Input: part model. Units: mm. Frame: model coordinates. Give positions to 0.01 mm unless a question says otherwise; leave off trailing zeros. Loops run counter-clockwise (first coordinate to the right, second up) from the corner with the lowest first, then second, coordinate; pieces in that order, holes last. Notation, with made-up numbers: M -40,76.5 L 17,76.5 A18 cw 17,110.5 Z; hole C -5.5,-29 d7. An arc over 180 degrees is marked long. Use CSV: the item, a comma, the result in double quotes. Start each with the question number.
from build123d import *

# Parameters (mm, degrees)
BOSS_EXTRU_1_DEPTH = 0.7


with BuildPart() as part:
    # Esquisse1 → Boss.-Extru.1 (new body)
    with BuildSketch(Plane.XY.offset(0.7)):
        with BuildLine():
            Line((0.632886418, 2.207137237), (0.815865574, 2.845261388))
            ThreePointArc((0.815865574, 2.845261388), (1.110405111, 3.18363768), (1.558931601, 3.174917521))
            ThreePointArc((1.558931601, 3.174917521), (2.501036685, 2.501036685), (3.174917521, 1.558931601))
            ThreePointArc((3.174917521, 1.558931601), (3.18363768, 1.110405111), (2.845261388, 0.815865574))
            Line((2.845261388, 0.815865574), (2.207137237, 0.632886418))
            ThreePointArc((2.207137237, 0.632886418), (2.027919172, 0.500132947), (1.979974043, 0.282316824))
            ThreePointArc((1.979974043, 0.282316824), (1.989252382, -0.2070627), (1.879385242, -0.684040287))
            Line((1.879385242, -0.684040287), (2.561408424, -2.557883579))
            ThreePointArc((2.561408424, -2.557883579), (3.113603209, -3.004615598), (3.76702433, -2.726174553))
            ThreePointArc((3.76702433, -2.726174553), (0, 4.65), (-3.76702433, -2.726174553))
            ThreePointArc((-3.76702433, -2.726174553), (-3.113603209, -3.004615598), (-2.561408424, -2.557883579))
            Line((-2.561408424, -2.557883579), (-1.879385242, -0.684040287))
            ThreePointArc((-1.879385242, -0.684040287), (-1.989252382, -0.2070627), (-1.979974043, 0.282316824))
            ThreePointArc((-1.979974043, 0.282316824), (-2.027919172, 0.500132947), (-2.207137237, 0.632886418))
            Line((-2.207137237, 0.632886418), (-2.845261388, 0.815865574))
            ThreePointArc((-2.845261388, 0.815865574), (-3.18363768, 1.110405111), (-3.174917521, 1.558931601))
            ThreePointArc((-3.174917521, 1.558931601), (-2.501036685, 2.501036685), (-1.558931601, 3.174917521))
            ThreePointArc((-1.558931601, 3.174917521), (-1.110405111, 3.18363768), (-0.815865574, 2.845261388))
            Line((-0.815865574, 2.845261388), (-0.632886418, 2.207137237))
            ThreePointArc((-0.632886418, 2.207137237), (-0.500132947, 2.027919172), (-0.282316824, 1.979974043))
            ThreePointArc((-0.282316824, 1.979974043), (0, 2), (0.282316824, 1.979974043))
            ThreePointArc((0.282316824, 1.979974043), (0.500132947, 2.027919172), (0.632886418, 2.207137237))
        make_face()
    extrude(amount=-BOSS_EXTRU_1_DEPTH)


solid = part.part
Item 1: Section B-B (x = -3). Output: boundary loops of the cut face in (y, z).
Item 2: First-contact query: pin 1 Ø2 at (x, y) = (0, 2.5) entering from -Z. Flat tip, straight axial feed; report the tip coordinate or a pass-through.
Item 3: Section C-C (z = 0.1). Output: boundary loops of the cut face in (x, y).
Item 4: Section A-A (y = 0). Output: boundary loops of the cut face in (x, z).
Item 5: Mould query, pull axis X, two halves, no side actions, for faces 1 (the cylindrical face through (0.143, 4.648, 0.355)), 2 (the cylindrical face through (-2.5, 2.5, 0.4)), 3 (the cylindrical face through (2.5, 2.5, 0.4)), 4 (the flat face through (0, 3, 0.7)). Classes: +X half, -X half, draft (parallel to the pull), parting line (faces both ways), or undercut.
Item 6: Material intervals for line 1 (X direction, y = 0, z = 0.55); line 2 (X direction, y = 2.5, z = 0.25); line 3 (X direction, y = -1, z = 0.1), sorted ascending.
Item 7: Section D-D (y = 3.5). Output: boundary loops of the cut face in (x, z), then the cut area to 3 significant figures.
Recorded:
1,outline,"M -2.98,0 L 0.89,0 L 0.89,0.7 L -2.98,0.7 Z; M 1.87,0 L 3.55,0 L 3.55,0.7 L 1.87,0.7 Z"
2,pin 1,"z = 0"
3,outline,"M -3.77,-2.73 A0.69 ccw -2.56,-2.56 L -1.88,-0.68 A2 cw -1.98,0.28 A0.32 ccw -2.21,0.63 L -2.85,0.82 A0.53 cw -3.17,1.56 A3.54 cw -1.56,3.17 A0.53 cw -0.82,2.85 L -0.63,2.21 A0.32 ccw -0.28,1.98 A2 cw 0.28,1.98 A0.32 ccw 0.63,2.21 L 0.82,2.85 A0.53 cw 1.56,3.17 A3.54 cw 3.17,1.56 A0.53 cw 2.85,0.82 L 2.21,0.63 A0.32 ccw 1.98,0.28 A2 cw 1.88,-0.68 L 2.56,-2.56 A0.69 ccw 3.77,-2.73 A4.65 ccw long Z"
4,outline,"M -4.65,0 L -2,0 L -2,0.7 L -4.65,0.7 Z; M 2,0 L 4.65,0 L 4.65,0.7 L 2,0.7 Z"
5,face 1,"parting line"
5,face 2,"undercut"
5,face 3,"undercut"
5,face 4,"draft"
6,line 1,"-4.65 to -2, 2 to 4.65"
6,line 2,"-3.92 to -2.5, -0.72 to 0.72, 2.5 to 3.92"
6,line 3,"-4.54 to -1.99, 1.99 to 4.54"
7,outline,"M -3.06,0 L 3.06,0 L 3.06,0.7 L -3.06,0.7 Z"
7,area,"4.29 mm²"
